from build123d import *

# Parameters (mm, degrees)
ESQUISSE1_W        = 80
ESQUISSE1_H        = 80
ESQUISSE1_R        = 2.5
BOSS_EXTRU_1_DEPTH = 2
ESQUISSE2_R        = 40
BOSS_EXTRU_2_DEPTH = 19
ESQUISSE3_R        = 21.5
BOSS_EXTRU_3_DEPTH = 2
CONG_1_R           = 5
CONG_2_R           = 2
CONG_3_R           = 1


with BuildPart() as part:
    # Esquisse1 → Boss.-Extru.1 (new body)
    with BuildSketch(Plane.XY):
        with Locations((5.633683954, -6.21564482)):
            Rectangle(ESQUISSE1_W, ESQUISSE1_H)
        with Locations((-30.337555091, 29.78435518)):
            Circle(ESQUISSE1_R, mode=Mode.SUBTRACT)
        with Locations((-30.337555091, -42.21564482)):
            Circle(ESQUISSE1_R, mode=Mode.SUBTRACT)
        with Locations(Location((41.604923, -42.21564482, 0), (0, 0, 180))):
            Circle(ESQUISSE1_R, mode=Mode.SUBTRACT)
        with Locations(Location((41.604923, 29.78435518, 0), (0, 0, 180))):
            Circle(ESQUISSE1_R, mode=Mode.SUBTRACT)
    extrude(amount=BOSS_EXTRU_1_DEPTH)

    # Esquisse2 → Boss.-Extru.2 (add)
    with BuildSketch(Plane.XY.offset(2)):
        with Locations((5.633683954, -6.21564482)):
            Circle(ESQUISSE2_R)
    extrude(amount=BOSS_EXTRU_2_DEPTH)

    # Esquisse3 → Boss.-Extru.3 (add)
    with BuildSketch(Plane.XY.offset(21)):
        with Locations((5.633683954, -6.21564482)):
            Circle(ESQUISSE3_R)
    extrude(amount=BOSS_EXTRU_3_DEPTH)

    # Congé1
    cong_1_edges = [part.edges().sort_by_distance(p)[0] for p in [
        (-34.366316046, 33.78435518, 1),
        (45.633683954, 33.78435518, 1),
        (45.633683954, -46.21564482, 1),
        (-34.366316046, -46.21564482, 1),
    ]]
    fillet(cong_1_edges, radius=CONG_1_R)

    # Congé2
    cong_2_edges = [part.edges().sort_by_distance(p)[0] for p in [
        (-15.866316046, -6.21564482, 23),
    ]]
    fillet(cong_2_edges, radius=CONG_2_R - 0.0001)  # a hair under: the kernel refuses the full size

    # Congé3
    cong_3_edges = [part.edges().sort_by_distance(p)[0] for p in [
        (-34.366316046, -6.21564482, 21),
    ]]
    fillet(cong_3_edges, radius=CONG_3_R)


solid = part.part
Here's how the part is built. I have some questions about the finished solid (model axes, mm). A direction names the side the tool comes from. Round coordinates to 2 decimals unless told otherwise and drop trailing zeros. Loops run counter-clockwise (first coordinate to the right, second up) from the corner with the lowest first, then second, coordinate; pieces in that order, holes last.
1. For P1, Ø2, axis at x = -19, y = -13.5, coming from the +Z side; P2, Ø6.5, axis at x = -30.34, y = 29.78, coming from the +Z side; P3, Ø3, axis at x = -30.34, y = -42.22, coming from the +Z side; P4, Ø10, axis at y = -13, z = 16.5, coming from the +X side, each with a flat end and sliding along its axis, tell me the tip position at first contact or that it passes through.
Answer list:
P1: stops at z = 21
P2: stops at z = 2
P3: passes through
P4: stops at x = 45.59
2. If we section it at A-A on z = 4.5: Write out the boundary of the cut face in (x, y), plus the area to 3 significant figures.
Answer list:
outline: circle Ø80 at (5.63, -6.22)
area: 5,030 mm2
3. If I drill on line 1 along Z through (x, y) = (36, 11); line 2 along Z through (x, y) = (-26.5, -40); line 3 along Y through (x, z) = (-13, 20.75), over which ranges is the centre line in solid material (lowest first)?
Answer list:
line 1: z = 0 to 21
line 2: z = 0 to 2
line 3: y = -41.23 to 28.8
4. Which directions (+Z, -Z, +X, -X, +Y, -Y) give clear straight access to the entire face, cutting with the end or side of a thin tool? Please do faces 1 (the face through (-3.038, -45.264, 10.874)), 2 (the face through (36, 24, 2)), 3 (the face through (45.634, -7, 1)), 4 (the face through (-25, -36, 2)), 5 (the face through (36, -36, 2)).
Answer list:
face 1: +Z
face 2: +Z, +X, +Y
face 3: +Z, -Z, +X, +Y, -Y
face 4: +Z, -X, -Y
face 5: +Z, +X, -Y
